from build123d import *

# Parameters (mm, degrees)
SKETCH1_W           = 25
SKETCH1_H           = 25
BOSS_EXTRUDE1_DEPTH = 2
FILLET1_R           = 3
CUT_EXTRUDE1_REACH  = 4
SKETCH2_R           = 1


with BuildPart() as part:
    # Sketch1 → Boss-Extrude1 (new body)
    with BuildSketch(Plane(origin=(0, 0, 0), x_dir=(1, 0, 0), z_dir=(0, 1, 0))):
        Rectangle(SKETCH1_W, SKETCH1_H)
    extrude(amount=BOSS_EXTRUDE1_DEPTH)

    # Fillet1
    fillet1_edges = [part.edges().sort_by_distance(p)[0] for p in [
        (12.5, 1, 12.5),
        (-12.5, 1, 12.5),
        (-12.5, 1, -12.5),
        (12.5, 1, -12.5),
    ]]
    fillet(fillet1_edges, radius=FILLET1_R)

    # Sketch2 → Cut-Extrude1 (cut, up to next)
    with BuildSketch(Plane(origin=(0, 2, 0), x_dir=(1, 0, 0), z_dir=(0, 1, 0)), mode=Mode.PRIVATE) as cut_extrude1_sk1:
        with Locations((-9.5, 9.5)):
            Circle(SKETCH2_R)
    cut_extrude1_tool1 = extrude(cut_extrude1_sk1.sketch, amount=-CUT_EXTRUDE1_REACH, mode=Mode.PRIVATE) & part.part
    add(cut_extrude1_tool1.solids().sort_by_distance((-9.5, 2, -9.5))[0], mode=Mode.SUBTRACT)
    # Sketch2 → Cut-Extrude1 (cut, up to next)
    with BuildSketch(Plane(origin=(0, 2, 0), x_dir=(1, 0, 0), z_dir=(0, 1, 0)), mode=Mode.PRIVATE) as cut_extrude1_sk2:
        with Locations((9.5, 9.5)):
            Circle(SKETCH2_R)
    cut_extrude1_tool2 = extrude(cut_extrude1_sk2.sketch, amount=-CUT_EXTRUDE1_REACH, mode=Mode.PRIVATE) & part.part
    add(cut_extrude1_tool2.solids().sort_by_distance((9.5, 2, -9.5))[0], mode=Mode.SUBTRACT)
    # Sketch2 → Cut-Extrude1 (cut, up to next)
    with BuildSketch(Plane(origin=(0, 2, 0), x_dir=(1, 0, 0), z_dir=(0, 1, 0)), mode=Mode.PRIVATE) as cut_extrude1_sk3:
        with Locations((9.5, -9.5)):
            Circle(SKETCH2_R)
    cut_extrude1_tool3 = extrude(cut_extrude1_sk3.sketch, amount=-CUT_EXTRUDE1_REACH, mode=Mode.PRIVATE) & part.part
    add(cut_extrude1_tool3.solids().sort_by_distance((9.5, 2, 9.5))[0], mode=Mode.SUBTRACT)
    # Sketch2 → Cut-Extrude1 (cut, up to next)
    with BuildSketch(Plane(origin=(0, 2, 0), x_dir=(1, 0, 0), z_dir=(0, 1, 0)), mode=Mode.PRIVATE) as cut_extrude1_sk4:
        with Locations((-9.5, -9.5)):
            Circle(SKETCH2_R)
    cut_extrude1_tool4 = extrude(cut_extrude1_sk4.sketch, amount=-CUT_EXTRUDE1_REACH, mode=Mode.PRIVATE) & part.part
    add(cut_extrude1_tool4.solids().sort_by_distance((-9.5, 2, 9.5))[0], mode=Mode.SUBTRACT)

    # Sketch3 → Revolve1 (revolve)
    with BuildSketch(Plane.XY):
        with BuildLine():
            Line((0, 2), (0, 4))
            ThreePointArc((0, 4), (1.505199322, 3.427724238), (2.25, 2))
            Line((2.25, 2), (0, 2))
        make_face()
    revolve(axis=Axis((0, 2, 0), (0, 1, 0)))


solid = part.part
CAD build for the part. Positions are in the model's coordinates, mm. Give positions to 0.01 mm unless a question says otherwise; leave off trailing zeros. Loops run counter-clockwise (first coordinate to the right, second up) from the corner with the lowest first, then second, coordinate; pieces in that order, holes last. Notation, with made-up numbers: M 48,39 L 54,39 A28 ccw 54,66 Z; hole C 51,64.5 d9. An arc over 180 degrees is marked long. Write each question's results on one line, items separated by ' | '.
Q1. Band-saw the part on B-B on x = -5. Write the cut outline in (y, z), and give its area (3 significant figures).
Geometry check:
outline: M 0,-12.5 L 2,-12.5 L 2,12.5 L 0,12.5 Z | area: 50.0 mm²
Q2. Band-saw the part on C-C on z = 3.25. Write the cut outline in (x, y).
Geometry check:
outline: M -12.5,0 L 12.5,0 L 12.5,2 L -12.5,2 Z
Q3. Band-saw the part on A-A on y = 0.4. Write the cut outline in (x, z), and give its area (3 significant figures).
Geometry check:
outline: M -12.5,-9.5 A3 ccw -9.5,-12.5 L 9.5,-12.5 A3 ccw 12.5,-9.5 L 12.5,9.5 A3 ccw 9.5,12.5 L -9.5,12.5 A3 ccw -12.5,9.5 Z; hole C -9.5,-9.5 d2; hole C -9.5,9.5 d2; hole C 9.5,-9.5 d2; hole C 9.5,9.5 d2 | area: 605 mm²
Q4. Flat gauge pins, fed straight in: P1, Ø1, axis at y = 3.5, z = 0.5, coming from the -X side; P2, Ø2.5, axis at x = -9.5, z = 9.5, coming from the +Y side; P3, Ø12.5, axis at x = 3.5, z = -5.5, coming from the +Y side. Where does each tip first touch, or does it go through?
Geometry check:
P1: stops at x = -1.83 | P2: stops at y = 2 | P3: stops at y = 3.98
Q5. Band-saw the part on D-D on y = 3.2. Write the cut outline in (x, z).
Geometry check:
outline: C 0,0 d3.46
Q6. Probe probe 1 along Z at (x, y) = (9.5, 0.65); probe 2 along Z at (x, y) = (-10, 0.55). List the from-to ranges inside material, lowest first.
Geometry check:
probe 1: z = -12.5 to -10.5, -8.5 to 8.5, 10.5 to 12.5 | probe 2: z = -12.46 to -10.37, -8.63 to 8.63, 10.37 to 12.46
Q7. Mould opens along X. For faces 1 (the face through (9.37, 1.01, 8.51)), 2 (the face through (12.5, 1, 0)), 3 (the face through (0, 1, 12.5)) say: pulls with the +X half, pulls with the -X half, needs draft (parallel to the pull), parting line crosses it, or undercut.
Geometry check:
face 1: undercut | face 2: pulls with the +X half | face 3: needs draft
